The model under review builds one solid part; all positions refer to its coordinate system, in mm. Coordinates: 2 decimals unless noted, no trailing zeros. Write each loop counter-clockwise with the first axis right and the second up, starting at its lowest first coordinate (ties: lowest second). Pieces come first, ordered by that corner, then holes. Notation, with made-up numbers: (-25, 52.5) - (15, 52.5) arc R21 cw to (15, 59.5) - close; hole circle Ø4 at (56.25, 58.5). An arc over 180 degrees is marked (long way). Use one line per item in the form item = value. Start each with the question number.
```python
from build123d import *

# Parameters (mm, degrees)
SKETCH3_W          = 228.6
SKETCH3_H          = 38.1
SKETCH3_R          = 2.54
SKETCH3_R_2        = 10.16
BASE_FLANGE1_DEPTH = 4.7625


# Sheet-metal steps are written as plain solids
with BuildPart() as part:
    # Sketch3 → Base-Flange1 (new body)
    with BuildSketch(Plane(origin=(0, 0, 0), x_dir=(1, 0, 0), z_dir=(0, 1, 0))):
        with Locations((-114.3, 0)):
            Rectangle(SKETCH3_W, SKETCH3_H)
        with Locations(Location((-220.98, 0, 0), (0, 0, 270))):
            Circle(SKETCH3_R, mode=Mode.SUBTRACT)
        with Locations(Location((-195.58, 0, 0), (0, 0, 270))):
            Circle(SKETCH3_R_2, mode=Mode.SUBTRACT)
        with Locations(Location((-170.18, 0, 0), (0, 0, 270))):
            Circle(SKETCH3_R, mode=Mode.SUBTRACT)
    extrude(amount=-BASE_FLANGE1_DEPTH)


solid = part.part
```
1. Take a section at A-A (x = -195.58). State the section outline as (y, z) points, plus the area to 3 significant figures.
2. For L1, parallel to X at y = -2.75, z = 0; L2, parallel to Z at x = -220.98, y = -1.3; L3, parallel to X at y = -2.5, z = 1, list the stretches that pass through material, from the lowest coordinate up.
3. Take a section at B-B (y = -1.05). State the section outline as (x, z) points.
4. The part is to be moulded in two halves that separate along X. For faces 1 (the cylindrical face through (-167.66, -2.35, -0.33)), 2 (the flat face through (-116, 0, 0)), 3 (the flat face through (0, -2, 0)), 4 (the cylindrical face through (-205.5, -2.3, -2.2)), say which applies: released by +X, released by -X, zero draft, split by the parting line, or undercut.
5. Take a section at C-C (z = -7). State the section outline as (x, y) points.
Returned:
q1.outline = (-4.76, -19.05) - (0, -19.05) - (0, -10.16) - (-4.76, -10.16) - close; (-4.76, 10.16) - (0, 10.16) - (0, 19.05) - (-4.76, 19.05) - close
q1.area = 84.7 mm²
q2.L1 = -228.6 to -223.52, -218.44 to -205.74, -185.42 to -172.72, -167.64 to 0
q2.L2 = -19.05 to -2.54, 2.54 to 19.05
q2.L3 = -228.6 to -223.31, -218.65 to -205.69, -185.47 to -172.51, -167.85 to 0
q3.outline = (-228.6, -19.05) - (0, -19.05) - (0, 19.05) - (-228.6, 19.05) - close; hole circle Ø5.08 at (-220.98, 0); hole circle Ø20.32 at (-195.58, 0); hole circle Ø5.08 at (-170.18, 0)
q4.face_1 = undercut
q4.face_2 = zero draft
q4.face_3 = released by +X
q4.face_4 = undercut
q5.outline = (-228.6, -4.76) - (-202.94, -4.76) - (-202.94, 0) - (-228.6, 0) - close; (-188.22, -4.76) - (0, -4.76) - (0, 0) - (-188.22, 0) - close
